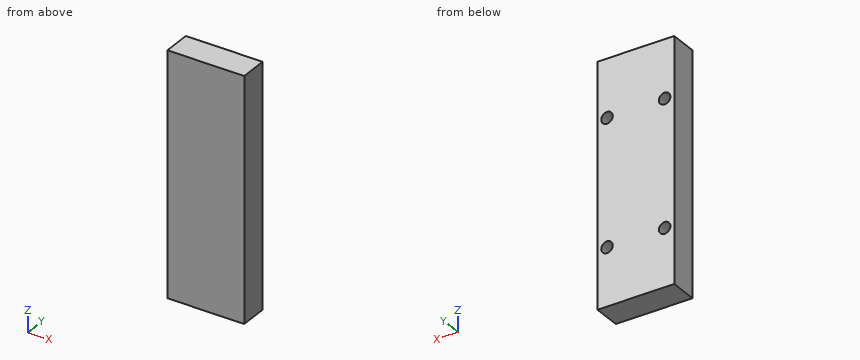
from build123d import *

# Parameters (mm, degrees)
SKETCH_1_W             = 22
SKETCH_1_H             = 8
EXTRUDE_1_DEPTH        = 69
HOLE_WIZARD_M4_1_D     = 3.3
HOLE_WIZARD_M4_1_DEPTH = 7
HOLE_WIZARD_M4_1_TIP   = 0.991420021


with BuildPart() as part:
    # 草图1 → 凸台-拉伸1 (new body)
    with BuildSketch(Plane.XY):
        Rectangle(SKETCH_1_W, SKETCH_1_H)
    extrude(amount=EXTRUDE_1_DEPTH)

    # M4 螺纹孔1
    with Locations(Plane(origin=(-8.25, 4, 16.5), x_dir=(0, 0, 1), z_dir=(0, 1, 0))):
        with Locations((0, 0), (0, 16.5), (36, 16.5), (36, 0)):
            Hole(HOLE_WIZARD_M4_1_D / 2, depth=HOLE_WIZARD_M4_1_DEPTH)
            with Locations((0, 0, -(HOLE_WIZARD_M4_1_DEPTH + HOLE_WIZARD_M4_1_TIP / 2))):  # 118° drill point
                Cone(0, HOLE_WIZARD_M4_1_D / 2, HOLE_WIZARD_M4_1_TIP, mode=Mode.SUBTRACT)


solid = part.part
The model under review builds one solid part; all positions refer to its coordinate system, in mm. Give positions to 0.01 mm unless a question says otherwise; leave off trailing zeros. Order: outer loops, then holes, each group sorted by start corner. A loop starts at its lowest first (then second) coordinate and runs counter-clockwise, first axis right, second up. Notation, with made-up numbers: (-21, 66) -> (3, 66) arc R18 ccw to (3, 82) -> close; hole circle Ø5 at (57, -24). An arc over 180 degrees is marked (long way). Write item = value, one per line. Start each with the question number.
(1) Take a section at A-A (y = -1.5). Write out the cut boundary in (x, z), plus the area to 3 significant figures.
(2) For L1, parallel to X at y = 1.5, z = 16.5; L2, parallel to Z at x = 8.25, y = -0.75; L3, parallel to Z at x = 8, y = -3.25, list the stretches that pass through material, from the lowest coordinate up. Write a range as from..to.
(3) For pin 1 Ø3 at (x, z) = (-8.25, 16.5) entering from +Y, flat-tipped, find the tip position at first contact; note if it passes through.
Returned:
q1.outline = (-11, 0) -> (11, 0) -> (11, 69) -> (-11, 69) -> close; hole circle Ø3.3 at (-8.25, 16.5); hole circle Ø3.3 at (-8.25, 52.5); hole circle Ø3.3 at (8.25, 16.5); hole circle Ø3.3 at (8.25, 52.5)
q1.area = 1,480 mm²
q2.L1 = -11..-9.9, -6.6..6.6, 9.9..11
q2.L2 = 0..14.85, 18.15..50.85, 54.15..69
q2.L3 = 0..15.29, 17.71..51.29, 53.71..69
q3.pin_1 = -3.09
